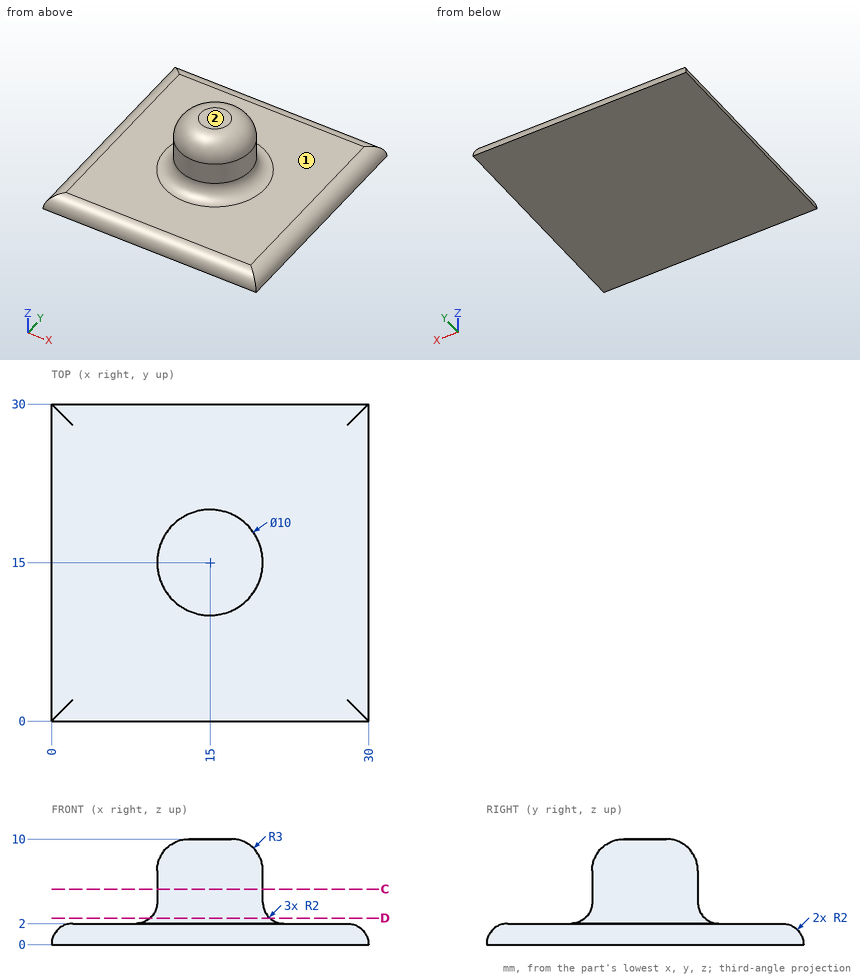
Part print with two shaded views. Sizes in mm from the minimum x, y, z corner. A direction names the side the tool comes from. Give positions to 0.01 mm unless a question says otherwise; leave off trailing zeros. Loops run counter-clockwise (first coordinate to the right, second up) from the corner with the lowest first, then second, coordinate; pieces in that order, holes last. Notation, with made-up numbers: (64.5, 71) - (110.5, 71) arc R15 ccw to (110.5, 99) - close; hole circle Ø3 at (-26, -35.5). An arc over 180 degrees is marked (long way). Put each result on its own line as item: value.
Q1. Slice it at C-C (z = 5.25). Give the cut face in (x, y), plus the area to 3 significant figures.
Filled in:
outline: circle Ø10 at (15, 15)
area: 78.5 mm²
Q2. Probe line 1 along Z through (x, y) = (23, 20); line 2 along Y through (x, z) = (7.25, 1.25); line 3 along Z through (x, y) = (1.5, 19.5). List the from-to ranges inside material, lowest first.
Filled in:
line 1: z = 0 to 2
line 2: y = 0.44 to 29.56
line 3: z = 0 to 1.94
Q3. Slice it at D-D (z = 2.5). Give the cut face in (x, y).
Filled in:
outline: circle Ø11.35 at (15, 15)
Q4. Tool access for the marked faces 1 and 2: list every direction of +Z, -Z, +X, -X, +Y, -Y with a clear straight run to the whole face (end or side of a thin tool).
Filled in:
face 1: +Z
face 2: +Z, +X, -X, +Y, -Y
